Source: CAD feature listing. Evaluate the final solid. Frame: model axes, mm. Face numbers are marked on the shaded views. A direction names the side the tool comes from. Coordinates: 2 decimals unless noted, no trailing zeros. Loops run counter-clockwise (first coordinate to the right, second up) from the corner with the lowest first, then second, coordinate; pieces in that order, holes last.
Item 1: Section query B-B, the plane x = 5.25. Return the cut outline in (y, z).
Item 2: Section query C-C, the plane z = -18. Return the cut outline in (x, y) (3 decimals).
Item 3: Section query D-D, the plane y = 17. Return the cut outline in (x, z), then the cut area to 3 significant figures.
Item 4: Line query: probe 1 along Z at (x, y) = (0.55, 5.5); probe 2 along Y at (x, z) = (1.1, -10); probe 3 along X at (y, z) = (28.5, -6). Output: solid intervals per line, ascending.
Item 5: Reachability of the marked faces 1, 2, 3 and 4 from +Z, -Z, +X, -X, +Y, -Y: full face, straight path, thin tool, end or side. Return the list, or none.
Item 6: Pin query (flat end, axial travel): pin 1 Ø1 at (x, z) = (5, -8.5) entering from -Y; pin 2 Ø1 at (y, z) = (25, -4.5) entering from -X; pin 3 Ø0.8 at (x, z) = (2, -9) entering from +Y (3 decimals); pin 4 Ø1.5 at (x, y) = (12.5, 20) entering from -Z (3 decimals). Return the tip coordinate at first contact, or that it passes through.
Item 7: Pull-direction query (Y, two-part tool) for the marked faces 5, 6 and 7; classes: +Y half, -Y half, draft (parallel to the pull), parting line (faces both ways), or undercut.
Item 8: Section query A-A, the plane z = -10. State how many separate pieces and enclosed holes the cut face has, then the cut area to 3 significant figures.
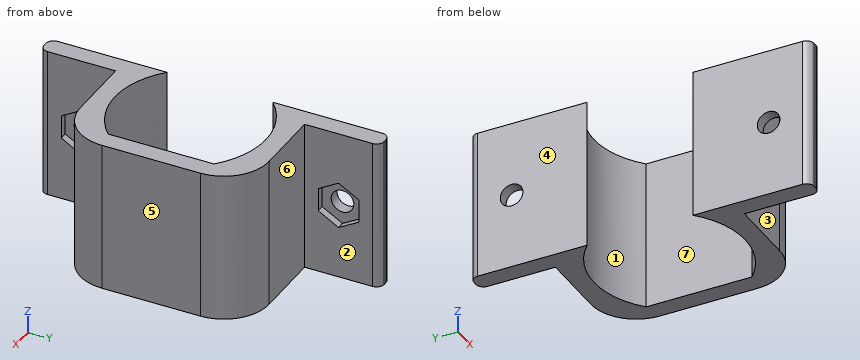
```python
from build123d import *

# Parameters (mm, degrees)
PAD_DEPTH            = 20
POCKET_DEPTH         = 20.001
FILLET_R             = 6
FILLET001_R          = 1
POCKET001_DEPTH      = 1
SKETCH003_R          = 1.5
POCKET002_DEPTH      = 1.501
BODY_PLACEMENT_ANGLE = 90


with BuildPart() as part:
    # Sketch → Pad (new body)
    with BuildSketch(Plane.YZ):
        Polygon((0, 0), (0, 2.5), (10, 2.5), (10, 17.5), (35, 17.5), (35, 2.5), (45, 2.5), (45, 0), align=None)
    extrude(amount=PAD_DEPTH)

    # Sketch001 (on Face10 of Pad) → Pocket (cut, through all)
    with BuildSketch(Plane.YZ.offset(20)):
        with BuildLine():
            Line((15.5, 15), (29.5, 15))
            ThreePointArc((29.5, 0), (32.5, 7.5), (29.5, 15))
            Line((15.5, 0), (29.5, 0))
            ThreePointArc((15.5, 15), (12.5, 7.5), (15.5, 0))
        make_face()
    extrude(amount=-POCKET_DEPTH, mode=Mode.SUBTRACT)

    # Fillet
    fillet_edges = [part.edges().sort_by_distance(p)[0] for p in [
        (10, 10, 17.5),
        (10, 35, 17.5),
    ]]
    fillet(fillet_edges, radius=FILLET_R)

    # Fillet001
    fillet001_edges = [part.edges().sort_by_distance(p)[0] for p in [
        (10, 0, 2.5),
        (10, 0, 0),
        (10, 45, 2.5),
        (10, 45, 0),
    ]]
    fillet(fillet001_edges, radius=FILLET001_R)

    # Sketch002 (on Face2 of Fillet001) → Pocket001 (cut)
    with BuildSketch(Plane(origin=(0, 0, 2.5), x_dir=(0, -1, 0), z_dir=(0, 0, 1))):
        Polygon((-36.815321, 11.55), (-39.5, 13.1), (-42.184679, 11.55), (-42.184679, 8.45), (-39.5, 6.9), (-36.815321, 8.45), align=None)
        Polygon((-2.815321, 8.45), (-2.815321, 11.55), (-5.5, 13.1), (-8.184679, 11.55), (-8.184679, 8.45), (-5.5, 6.9), align=None)
    extrude(amount=-POCKET001_DEPTH, mode=Mode.SUBTRACT)

    # Sketch003 (on Face33 of Pocket001) → Pocket002 (cut, through all)
    with BuildSketch(Plane(origin=(0, 0, 1.5), x_dir=(0, -1, 0), z_dir=(0, 0, 1))):
        with Locations((-39.5, 10)):
            Circle(SKETCH003_R)
        with Locations((-5.5, 10)):
            Circle(SKETCH003_R)
    extrude(amount=-POCKET002_DEPTH, mode=Mode.SUBTRACT)


with BuildPart() as part_1:
    # Body placement: moved
    add(part.part.rotate(Axis((0, 0, 0), (0, 1, 0)), BODY_PLACEMENT_ANGLE))


solid = part_1.part
```
Verdict:
1. outline: (10, -20) - (12.74, -20) - (12.74, 0) - (10, 0) - close; (32.26, -20) - (35, -20) - (35, 0) - (32.26, 0) - close
2. outline: (0, 1) arc R1 ccw to (1, 0) - (1.5, 0) arc R1 ccw to (2.5, 1) - (2.5, 10) - (11.5, 10) arc R6 ccw to (17.5, 16) - (17.5, 29) arc R6 ccw to (11.5, 35) - (2.5, 35) - (2.5, 44) arc R1 ccw to (1.5, 45) - (1, 45) arc R1 ccw to (0, 44) - (0, 29.5) arc R10.875 cw to (15, 29.5) - (15, 15.5) arc R10.875 cw to (0, 15.5) - close
3. outline: (15, -20) - (17.5, -20) - (17.5, 0) - (15, 0) - close
3. area: 50.0 mm2
4. probe 1: z = -20 to -11.5, -8.5 to 0
4. probe 2: y = 0 to 4, 7 to 14.58, 30.42 to 38, 41 to 45
4. probe 3: x = 15 to 17.5
5. face 1: +Z, -Z
5. face 2: +Z, -Z, +X, +Y
5. face 3: +Z, -Z, +X, -Y
5. face 4: +Z, -Z, -X, +Y, -Y
6. pin 1: stops at y = 10
6. pin 2: stops at x = 15
6. pin 3: stops at y = 44.995
6. pin 4: passes through
7. face 5: draft
7. face 6: +Y half
7. face 7: undercut
8. separate pieces: 3
8. enclosed holes: 0
8. area: 180 mm2
